Geometry check sheet. Reference: the model listing, model coordinates, mm. Coordinates: 2 decimals unless noted, no trailing zeros. Write each loop counter-clockwise with the first axis right and the second up, starting at its lowest first coordinate (ties: lowest second). Pieces come first, ordered by that corner, then holes. Notation, with made-up numbers: M 78.25,32.5 L 110.25,32.5 A17 cw 110.25,48.5 Z; hole C 32.5,35.5 d2. An arc over 180 degrees is marked long. Answer as a JSON object with one key per item and string values. Group by question number.
```python
from build123d import *

# Parameters (mm, degrees)
F0_R     = 2.5
F0_R_2   = 1.5
F0_R_3   = 5.75
F0_R_4   = 11.8
F1_DEPTH = 3


with BuildPart() as f1:
    # F0 (on Top) → F1 (new body)
    with BuildSketch(Plane.XY):
        Polygon((100, 35), (0, 35), (0, 0), (100.10055, 0), align=None)
        with Locations((4.89945, 5)):
            Circle(F0_R, mode=Mode.SUBTRACT)
        with Locations((79.588087, 5.5)):
            Circle(F0_R_2, mode=Mode.SUBTRACT)
        with Locations((95.10055, 5)):
            Circle(F0_R, mode=Mode.SUBTRACT)
        with Locations((22.599816, 17.507559)):
            Circle(F0_R_3, mode=Mode.SUBTRACT)
        with Locations((4.89945, 30)):
            Circle(F0_R, mode=Mode.SUBTRACT)
        with Locations((70.088087, 17.5)):
            Circle(F0_R_4, mode=Mode.SUBTRACT)
        with Locations((60.537812, 29.5)):
            Circle(F0_R_2, mode=Mode.SUBTRACT)
        with Locations((95.10055, 30)):
            Circle(F0_R, mode=Mode.SUBTRACT)
    extrude(amount=F1_DEPTH)


solid = f1.part
```
1) Section check D-D (y = 24.5). Record the cut outline in (x, z).
2) Material ranges on probe 1 along Y at (x, z) = (5, 1.9); probe 2 along X at (y, z) = (18, 1.1); probe 3 along Y at (x, z) = (60.5, 1.8), recorded low to high. Write a range as [from, to].
3) Section check A-A (x = 80). Record the cut outline in (y, z).
4) Section check B-B (y = 8.5). Record the cut outline in (x, z), then the cut area to 3 significant figures.
5) Go/stop test with a flat-tipped pin: pin 1 Ø9 at (x, y) = (22.6, 17.51) entering from -Z. Record where the tip stops, or that it passes through.
6) Section check C-C (z = 1.6). State how many separate pieces and enclosed holes the cut face has, then the cut area to 3 significant figures.
7) Draft check along X on faces 1 (the flat face through (0, 18, 1)), 2 (the flat face through (49, 18, 0)), 3 (the cylindrical face through (25.253, 12.406, 1.479)). Enter one of: +X half, -X half, draft (parallel to the pull), parting line (faces both ways), or undercut.
Entries:
{
 "1": {"outline": "M 0,0 L 60.59,0 L 60.59,3 L 0,3 Z; M 79.59,0 L 100.03,0 L 100.03,3 L 79.59,3 Z"},
 "2": {"probe 1": "[0, 2.5], [7.5, 27.5], [32.5, 35]", "probe 2": "[0, 16.87], [28.33, 58.3], [81.88, 100.05]", "probe 3": "[0, 10.62], [24.38, 28], [31, 35]"},
 "3": {"outline": "M 0,0 L 4.06,0 L 4.06,3 L 0,3 Z; M 6.94,0 L 11.1,0 L 11.1,3 L 6.94,3 Z; M 23.9,0 L 35,0 L 35,3 L 23.9,3 Z"},
 "4": {"outline": "M 0,0 L 62.46,0 L 62.46,3 L 0,3 Z; M 77.72,0 L 100.08,0 L 100.08,3 L 77.72,3 Z", "area": "254 mm^2"},
 "5": {"pin 1": "through"},
 "6": {"separate pieces": "1", "enclosed holes": "8", "area": "2,870 mm^2"},
 "7": {"face 1": "-X half", "face 2": "draft", "face 3": "undercut"}
}
